Can you work these out from the model? Positions are in its coordinate system, mm. Face numbers are marked on the shaded views. A direction names the side the tool comes from. Coordinates: 2 decimals unless noted, no trailing zeros. Order: outer loops, then holes, each group sorted by start corner. A loop starts at its lowest first (then second) coordinate and runs counter-clockwise, first axis right, second up. Notation, with made-up numbers: (15.5, 1.5) - (51.5, 1.5) arc R20 cw to (51.5, 21.5) - close; hole circle Ø11 at (71.5, 30.25). An arc over 180 degrees is marked (long way). Return JSON: item names as keys, results as strings. Group by question number.
1) Imagine slicing it at D-D (x = 16). Write out the boundary of the cut face in (y, z).
2) Imagine slicing it at C-C (x = -11.5). Write out the boundary of the cut face in (y, z).
3) If I drill on line 1 along Y through (x, z) = (11.5, -7.25); line 2 along X through (y, z) = (11.5, -1.75); line 3 along X through (y, z) = (11.5, -6.25), over which ranges is the centre line in solid material (lowest first)?
4) Imagine slicing it at A-A (z = -12.5). Give the number of separate pieces and of enclosed holes in the cut face, and give its area (3 significant figures).
5) If we mould it in two halves opening along X, with no side actions, what happens to the marked faces 1, 2 and 3? For each: pulls with the +X half, pulls with the -X half, needs draft (parallel to the pull), parting line crosses it, or undercut.
6) Which directions (+Z, -Z, +X, -X, +Y, -Y) give clear straight access to the entire face, cutting with the end or side of a thin tool? Please do the marked faces 4, 5, 6, 7 and 8.
7) For pin 1 Ø4.5 at (x, z) = (20, -12.5) entering from +Y; pin 2 Ø8.5 at (x, y) = (-2, -3) entering from -Z; pin 3 Ø7.5 at (y, z) = (8, -4) entering from -X; pin 4 Ø2 at (x, z) = (-20, -12.5) entering from -Y, each with a flat end and sliding along its axis, tell me the tip position at first contact or that it passes through.
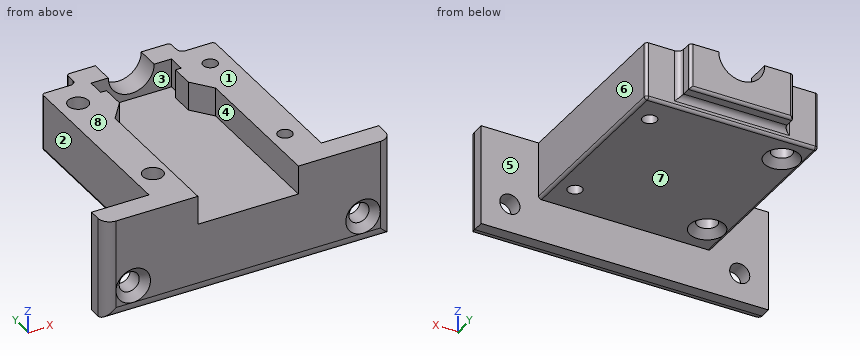
Solid Edge part; units mm, degrees
sketch "Sketch1" plane through (0, 0, 0) normal (0, -1, 0) x (1, 0, 0)
  line L0 (-15, 10) -> (15, 10)
  line L1 (15, 10) -> (15, -10)
  line L2 (15, -10) -> (-15, -10)
  line L3 (-15, -10) -> (-15, 10)
  dimension "D1" = 15
  dimension "D2" = 15
extrude "Protrusion1" add sketch "Sketch1" along normal mid plane 33
sketch "Sketch2" plane through (0, -16.5, 0) normal (0, -1, 0) x (1, 0, 0)
  line L0 (-25, 17.5) -> (25, 17.5)
  line L1 (25, 17.5) -> (25, -17.5)
  line L2 (25, -17.5) -> (-25, -17.5)
  line L3 (-25, -17.5) -> (-25, 17.5)
  dimension "D1" = 25
  dimension "D2" = 25
extrude "Ausprägung_2" add sketch "Sketch2" along normal blind 4
sketch "Sketch3" plane through (0, -20.5, 0) normal (0, -1, 0) x (1, 0, 0)
  line L0 (-8.75, 5) -> (8.75, 5)
  line L1 (8.75, 5) -> (8.75, -5)
  line L2 (8.75, -5) -> (-8.75, -5)
  line L3 (-8.75, -5) -> (-8.75, 5)
  dimension "D1" = 8.75
  dimension "D2" = 8.75
extrude "Ausschnitt_1" cut sketch "Sketch3" against normal blind 9
sketch "Sketch4" plane through (0, -11.5, 0) normal (0, -1, 0) x (1, 0, 0)
  line L0 (-8.75, 5) -> (8.75, 5)
  line L1 (8.75, 5) -> (8.75, -5)
  line L2 (8.75, -5) -> (-8.75, -5)
  line L3 (-8.75, -5) -> (-8.75, 5)
  dimension "D1" = 8.75
  dimension "D2" = 8.75
extrude "Ausschnitt_2" cut sketch "Sketch4" against normal blind 20
sketch "Sketch5" plane through (0, 16.5, 0) normal (0, 1, 0) x (-1, 0, 0)
  line L0 (6, 5) -> (6, -5)
  line L1 (6, -5) -> (-6, -5)
  line L2 (-6, -5) -> (-6, 5)
  line L3 (-6, 5) -> (6, 5)
  dimension "D1" = 6
  dimension "D2" = 6
extrude "Ausschnitt_3" cut sketch "Sketch5" against normal blind 8
sketch "Sketch6" plane through (0, -20.5, 0) normal (0, -1, 0) x (1, 0, 0)
  line L0 (-37.3753, 23.8002) -> (37.3753, 23.8002)
  line L1 (37.3753, 23.8002) -> (37.3753, 0)
  line L2 (37.3753, 0) -> (-37.3753, 0)
  line L3 (-37.3753, 0) -> (-37.3753, 23.8002)
extrude "Ausschnitt_4" cut sketch "Sketch6" against normal blind 187.325
hole "Bohrung_1" at (20, -20.5, -12.5) direction (0, 1, 0) diameter 3.5 end up to next countersink diameter 6 countersink angle 90
hole "Hole1" at (-20, -20.5, -12.5) direction (0, 1, 0) diameter 3.5 end up to next countersink diameter 6 countersink angle 90
hole "Bohrung_3" at (11.5, -11.5, 0) direction (0, 0, -1) diameter 2.5 end through all
hole "Hole2" at (11.5, 11.5, 0) direction (0, 0, -1) diameter 2.5 end through all
hole "Bohrung_5" at (-11.5, 11.5, -10) direction (0, 0, 1) diameter 3.5 end up to next countersink diameter 6 countersink angle 90
hole "Hole3" at (-11.5, -11.5, -10) direction (0, 0, 1) diameter 3.5 end up to next countersink diameter 6 countersink angle 90
fillet "Verrundung_2" radius 2 3 edges at (25, -20.5, -8.75) (0, -20.5, -17.5) (-25, -20.5, -8.75)
fillet "Verrundung_3" radius 0.5 5 edges at (15, 0, -10) (0, 16.5, -10) (-15, 0, -10) (-15, 16.5, -5) (15, 16.5, -5)
sketch "Sketch7" plane through (-15.5, -2, 0) normal (0, 0, 1) x (1, 0, 0)
  line L0 (8.5, 17.5) -> (9.5, 17.5)
  line L1 (9.5, 17.5) -> (9.5, 14.5)
  line L2 (9.5, 14.5) -> (8.5, 14.5)
  line L3 (8.5, 14.5) -> (8.5, 17.5)
  dimension "D1" = 8.5
  dimension "D2" = 8.5
extrude "Ausschnitt_6" cut sketch "Sketch7" against normal blind 5
sketch "Sketch8" plane through (15.5, -2, 0) normal (0, 0, 1) x (1, 0, 0)
  line L0 (-9.5, 17.5) -> (-8.5, 17.5)
  line L1 (-8.5, 17.5) -> (-8.5, 14.5)
  line L2 (-8.5, 14.5) -> (-9.5, 14.5)
  line L3 (-9.5, 14.5) -> (-9.5, 17.5)
  dimension "D1" = 8.5
  dimension "D2" = 9.5
extrude "Ausschnitt_7" cut sketch "Sketch8" against normal blind 5
sketch "Sketch9" plane through (0, 16.5, -4.75) normal (0, 1, 0) x (1, 0, 0)
  line L0 (-9, 3.25) -> (-6, 3.25)
  line L1 (-6, 3.25) -> (-6, -4.75)
  line L2 (-6, -4.75) -> (-9, -4.75)
  line L3 (-9, -4.75) -> (-9, 3.25)
  dimension "D1" = 9
  dimension "D2" = 9
extrude "Ausprägung_3" add sketch "Sketch9" along normal blind 3
sketch "Sketch10" plane through (0, 16.5, -4.75) normal (0, 1, 0) x (1, 0, 0)
  line L0 (6, 3.25) -> (9, 3.25)
  line L1 (9, 3.25) -> (9, -4.75)
  line L2 (9, -4.75) -> (6, -4.75)
  line L3 (6, -4.75) -> (6, 3.25)
  dimension "D1" = 6
  dimension "D2" = 9
extrude "Ausprägung_4" add sketch "Sketch10" along normal blind 3
sketch "Sketch11" plane through (0, 16.5, -4.75) normal (0, 1, 0) x (1, 0, 0)
  line L0 (-6, 3.25) -> (6, 3.25)
  line L1 (6, 3.25) -> (6, 0.25)
  line L2 (6, 0.25) -> (-6, 0.25)
  line L3 (-6, 0.25) -> (-6, 3.25)
  dimension "D1" = 6
  dimension "D2" = 6
extrude "Ausprägung_5" add sketch "Sketch11" along normal blind 3
fillet "Verrundung_4" radius 1 3 edges at (0, 16.5, -8) (-9, 16.5, -4) (9, 16.5, -4)
fillet "Verrundung_5" radius 0.5 3 edges at (0, 19.5, -8) (-9, 19.5, -4) (9, 19.5, -4)
sketch "Sketch12" plane through (0, -0.5, -5) normal (0, 0, 1) x (0, -1, 0)
  line L0 (-9, 8.75) -> (-5.5, 8.75)
  line L1 (-5.5, 8.75) -> (-9, 6)
  line L2 (-9, 6) -> (-9, 8.75)
  dimension "D1" = 9
extrude "Ausprägung_6" add sketch "Sketch12" along normal blind 5
sketch "Sketch13" plane through (0, -0.5, -5) normal (0, 0, 1) x (0, -1, 0)
  line L0 (-9, -8.75) -> (-5.5, -8.75)
  line L1 (-5.5, -8.75) -> (-9, -6)
  line L2 (-9, -6) -> (-9, -8.75)
  dimension "D1" = 9
extrude "Ausprägung_7" add sketch "Sketch13" along normal blind 5
sketch "Sketch14" plane through (0, -0.5, -5) normal (0, 0, 1) x (0, -1, 0)
  line L0 (-20, 6) -> (-16, 6)
  line L1 (-16, 6) -> (-16, -6)
  line L2 (-16, -6) -> (-20, -6)
  line L3 (-20, -6) -> (-20, 6)
  dimension "D1" = 20
extrude "Ausprägung_9" add sketch "Sketch14" along normal blind 10
hole "Bohrung_7" at (0, 19.5, 0) direction (0, -1, 0) diameter 8 end up to next
sketch "Sketch15" plane through (0, 19.5, -1.25) normal (0, 1, 0) x (0, 0, 1)
  line L0 (1.25, 6) -> (6.25, 6)
  line L1 (6.25, 6) -> (6.25, -6)
  line L2 (6.25, -6) -> (1.25, -6)
  line L3 (1.25, -6) -> (1.25, 6)
extrude "Ausschnitt_8" cut sketch "Sketch15" against normal blind 244.475
Calculated:
{
 "1": {"outline": "(-20.5, -15.5) arc R2 ccw to (-18.5, -17.5) - (-16.5, -17.5) - (-16.5, 0) - (-20.5, 0) - close"},
 "2": {"outline": "(-20.5, -15.5) arc R2 ccw to (-18.5, -17.5) - (-16.5, -17.5) - (-16.5, -10) - (-14.5, -10) - (-13.25, -8.75) - (-13.25, 0) - (-20.5, 0) - close; (-9.75, -8.75) - (-8.5, -10) - (8.5, -10) - (9.75, -8.75) - (9.75, 0) - (-9.75, 0) - close; (13.25, -8.75) - (14.5, -10) - (16, -10) arc R0.5 ccw to (16.5, -9.5) - (16.5, 0) - (13.25, 0) - close"},
 "3": {"line 1": "-20.5 to -12.75, -10.25 to 10.25, 12.75 to 16.5", "line 2": "-15 to -13.25, -9.75 to -6, 6 to 10.25, 12.75 to 15", "line 3": "-15 to -13.25, -9.75 to 10.25, 12.75 to 15"},
 "4": {"separate pieces": "3", "enclosed holes": "0", "area": "167 mm2"},
 "5": {"face 1": "needs draft", "face 2": "pulls with the -X half", "face 3": "undercut"},
 "6": {"face 4": "+Z, -Y", "face 5": "-Z, +Y", "face 6": "+Z, -Z, +X, +Y", "face 7": "-Z, +X, -X, +Y", "face 8": "+Z, +X, -X, +Y, -Y"},
 "7": {"pin 1": "y = -16.5", "pin 2": "z = -10", "pin 3": "x = -15", "pin 4": "through"}
}
